The model under review builds one solid part; all positions refer to its coordinate system, in mm. A direction names the side the tool comes from. Coordinates: 2 decimals unless noted, no trailing zeros. Loops run counter-clockwise (first coordinate to the right, second up) from the corner with the lowest first, then second, coordinate; pieces in that order, holes last. Notation, with made-up numbers: (55, 42.25) - (104, 42.25) arc R23 ccw to (104, 63.25) - close; hole circle Ø3 at (76, 68.5). An arc over 180 degrees is marked (long way). Answer in a Markdown table with one row per item. Add a question column.
(1) For P1, Ø3.5, axis at x = 5.66, z = 15.16, coming from the -Y side; P2, Ø10.5, axis at y = 19, z = -4.5, coming from the +X side; P3, Ø14.5, axis at y = 29.5, z = 2, coming from the +X side, all flat-tipped, find the tip position at first contact; note any pin that passes through.
(2) We need section C-C on z = 12. Write out the cut boundary in (x, y), plus the area to 3 significant figures.
(3) For line 1 along Z through (x, y) = (0, 33.5); line 2 along X through (y, z) = (26, -4); line 3 along Y through (x, z) = (18.5, -14.3), list the stretches that pass through material, from the lowest coordinate up.
(4) Machinability: for faces 5 (the flat face through (0, 20, -17.5)), 6 (the flat face through (12.5, 25, -4)), which of the approach directions +Z, -Z, +X, -X, +Y, -Y give a long, thin tool a straight path to every point of the face, cutting with its end or side? Answer none if there is none.
(5) We need section B-B on y = 27. Write out the cut boundary in (x, z), plus the area to 3 significant figures.
(6) Mouldability with a two-part tool opening along Y and no side actions: class faces 1 (the cylindrical face through (16, 7, -14)), 2 (the cylindrical face through (-21, 7, -14)), 3 (the flat face through (0, 0, -15)), 4 (the flat face through (-11.714, 32.134, 7.605)) as +Y half, -Y half, draft (parallel to the pull), parting line (faces both ways), or undercut.
(7) We need section D-D on y = 18. Write out the cut boundary in (x, z), plus the area to 3 significant figures.
(8) We need section A-A on x = 0. Write out the cut boundary in (y, z), plus the area to 3 significant figures.
from build123d import *

# Parameters (mm, degrees)
SKETCH_1_W           = 49
SKETCH_1_H           = 35
EXTRUDE_1_DEPTH      = 40
SKETCH_2_R           = 5
SKETCH_2_R_2         = 1.5
CUT_EXTRUDE_1_DEPTH  = 40
SKETCH_3_W           = 12
SKETCH_3_H           = 34
CUT_EXTRUDE_3_DEPTH  = 29
CUT_EXTRUDE_6_DEPTH  = 50
SKETCH_7_W           = 21
SKETCH_7_H           = 28.5
CUT_EXTRUDE_8_DEPTH  = 29
CUT_EXTRUDE_10_DEPTH = 29
SKETCH_12_R          = 2.5
CUT_EXTRUDE_12_DEPTH = 56.14752941
FILLET_1_R           = 10
FILLET_2_R           = 10
FILLET_4_R           = 3
EXTRUDE_2_DEPTH      = 11.5


with BuildPart() as part:
    # 草圖1 → 填料-伸長1 (new body)
    with BuildSketch(Plane(origin=(0, 0, 0), x_dir=(1, 0, 0), z_dir=(0, 1, 0))):
        Rectangle(SKETCH_1_W, SKETCH_1_H)
    extrude(amount=EXTRUDE_1_DEPTH)

    # 草圖2 → 除料-伸長1 (cut)
    with BuildSketch(Plane(origin=(0, 40, 0), x_dir=(1, 0, 0), z_dir=(0, 1, 0))):
        with Locations(Location((0, -9.5, 0), (0, 0, 270))):
            Circle(SKETCH_2_R)
        with Locations(Location((5.656854249, -3.843145751, 0), (0, 0, 270))):
            Circle(SKETCH_2_R_2)
        with Locations(Location((5.656854249, -15.156854249, 0), (0, 0, 90))):
            Circle(SKETCH_2_R_2)
        with Locations(Location((-5.656854249, -15.156854249, 0), (0, 0, 270))):
            Circle(SKETCH_2_R_2)
        with Locations(Location((-5.656854249, -3.843145751, 0), (0, 0, 90))):
            Circle(SKETCH_2_R_2)
    extrude(amount=-CUT_EXTRUDE_1_DEPTH, mode=Mode.SUBTRACT)

    # 草圖3 → 除料-伸長3 (cut)
    with BuildSketch(Plane.XY.offset(17.5)):
        with Locations((-18.5, 17)):
            Rectangle(SKETCH_3_W, SKETCH_3_H)
        with Locations((18.5, 17)):
            Rectangle(SKETCH_3_W, SKETCH_3_H)
    extrude(amount=-CUT_EXTRUDE_3_DEPTH, mode=Mode.SUBTRACT)

    # 草圖6 → 除料-伸長6 (cut)
    with BuildSketch(Plane(origin=(0, 40, 0), x_dir=(1, 0, 0), z_dir=(0, 1, 0))):
        with BuildLine():
            Line((-10.444900063, -9.5), (-24.5, 11.5))
            Line((-24.5, 11.5), (-24.5, -17.5))
            Line((-24.5, -17.5), (-6.715350871, -17.5))
            ThreePointArc((-6.715350871, -17.5), (-9.466707613, -13.913318966), (-10.444900063, -9.5))
        make_face()
        with BuildLine():
            Line((24.5, 11.5), (10.444900063, -9.5))
            ThreePointArc((10.444900063, -9.5), (9.466707613, -13.913318966), (6.715350871, -17.5))
            Line((6.715350871, -17.5), (24.5, -17.5))
            Line((24.5, -17.5), (24.5, 11.5))
        make_face()
    extrude(amount=-CUT_EXTRUDE_6_DEPTH, mode=Mode.SUBTRACT)

    # 草圖7 → 除料-伸長8 (cut)
    with BuildSketch(Plane.XY.offset(17.5)):
        with Locations((0, 14.25)):
            Rectangle(SKETCH_7_W, SKETCH_7_H)
    extrude(amount=-CUT_EXTRUDE_8_DEPTH, mode=Mode.SUBTRACT)

    # 草圖10 → 除料-伸長10 (cut)
    with BuildSketch(Plane.ZY.offset(12.5)):
        Polygon((-11.5, 0), (6.429434947, 0), (9.417674105, 0), (9.417674105, 28.5), (-11.5, 7.582325895), align=None)
    extrude(amount=-CUT_EXTRUDE_10_DEPTH, mode=Mode.SUBTRACT)

    # 草圖12 → 除料-伸長12 (cut, through all)
    with BuildSketch(Plane.XY.offset(-11.5)):
        with Locations((18.5, 7)):
            Circle(SKETCH_12_R)
        with Locations((18.5, 27)):
            Circle(SKETCH_12_R)
        with Locations((-18.5, 7)):
            Circle(SKETCH_12_R)
        with Locations((-18.5, 27)):
            Circle(SKETCH_12_R)
    extrude(amount=-CUT_EXTRUDE_12_DEPTH, mode=Mode.SUBTRACT)

    # 圓角1
    fillet_1_edges = [part.edges().sort_by_distance(p)[0] for p in [
        (-24.5, 0, -14.5),
    ]]
    fillet(fillet_1_edges, radius=FILLET_1_R)

    # 圓角2
    fillet_2_edges = [part.edges().sort_by_distance(p)[0] for p in [
        (24.5, 0, -14.5),
    ]]
    fillet(fillet_2_edges, radius=FILLET_2_R)

    # 圓角4
    fillet_4_edges = [part.edges().sort_by_distance(p)[0] for p in [
        (-18.5, 34, -2.535282526),
        (-17.472450031, 40, -1),
        (17.472450031, 40, -1),
        (18.5, 34, -2.535282526),
    ]]
    fillet(fillet_4_edges, radius=FILLET_4_R - 0.0001)  # a hair under: the kernel refuses the full size

    # 草圖14 → 填料-伸長2 (add)
    with BuildSketch(Plane(origin=(0, 40, 0), x_dir=(1, 0, 0), z_dir=(0, 1, 0))):
        with BuildLine():
            Line((-6.715350871, -17.5), (6.715350871, -17.5))
            ThreePointArc((6.715350871, -17.5), (0, -20.281589407), (-6.715350871, -17.5))
        make_face()
    extrude(amount=-EXTRUDE_2_DEPTH)


solid = part.part
Outcome:
| question | item | result |
|---|---|---|
| 1 | P1 | y = 28.5 |
| 1 | P2 | x = 12.5 |
| 1 | P3 | x = 17.74 |
| 2 | outline | (-10.14, 28.5) - (-4.33, 28.5) - (-4.33, 40) - (-10.14, 40) - close; (4.33, 28.5) - (10.14, 28.5) - (10.14, 40) - (4.33, 40) - close |
| 2 | area | 134 mm² |
| 3 | line 1 | -17.5 to 4.5, 14.5 to 20.28 |
| 3 | line 2 | -12.5 to -10.5, 10.5 to 12.5 |
| 3 | line 3 | 0.83 to 4.5, 9.5 to 24.5, 29.5 to 40 |
| 4 | face 5 | -Z, +X, -X, +Y, -Y |
| 4 | face 6 | +Z, +X, -Y |
| 5 | outline | (-24.5, -17.5) - (-21, -17.5) - (-21, -11.5) - (-24.5, -11.5) - close; (-16, -17.5) - (16, -17.5) - (16, -11.5) - (12.5, -11.5) - (12.5, 6.43) - (11.5, 7.92) - (10.5, 7.92) - (10.5, -11.5) - (-10.5, -11.5) - (-10.5, 7.92) - (-11.5, 7.92) - (-12.5, 6.43) - (-12.5, -11.5) - (-16, -11.5) - close; (21, -17.5) - (24.5, -17.5) - (24.5, -11.5) - (21, -11.5) - close |
| 5 | area | 310 mm² |
| 6 | face 1 | undercut |
| 6 | face 2 | undercut |
| 6 | face 3 | -Y half |
| 6 | face 4 | draft |
| 7 | outline | (-24.5, -17.5) - (24.5, -17.5) - (24.5, -11.5) - (12.5, -11.5) - (12.5, -1.08) - (10.5, -1.08) - (10.5, -11.5) - (-10.5, -11.5) - (-10.5, -1.08) - (-12.5, -1.08) - (-12.5, -11.5) - (-24.5, -11.5) - close |
| 7 | area | 336 mm² |
| 8 | outline | (0, -17.5) - (40, -17.5) - (40, 4.5) - (28.5, 4.5) - (28.5, -11.5) - (0, -11.5) - close; (28.5, 14.5) - (40, 14.5) - (40, 20.28) - (28.5, 20.28) - close |
| 8 | area | 490 mm² |
